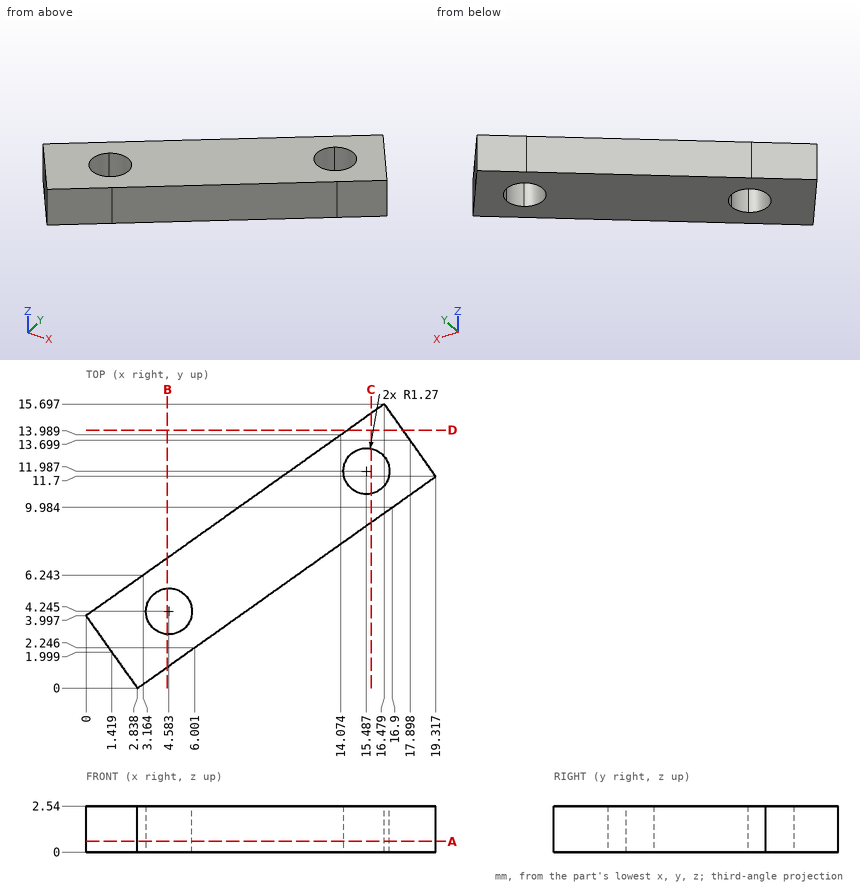
Geometry: see drawing. Coordinates: mm, zero at the bounding-box minimum. Give positions to 0.01 mm unless a question says otherwise; leave off trailing zeros. Loops run counter-clockwise (first coordinate to the right, second up) from the corner with the lowest first, then second, coordinate; pieces in that order, holes last. Notation, with made-up numbers: (-16, -19) - (33, -19) arc R20 ccw to (33, 7) - close; hole circle Ø7 at (31.25, -12). An arc over 180 degrees is marked (long way). Use CSV: the item, a comma, the result in double quotes. Start each with the question number.
1. Pin query (flat end, axial travel): pin 1 (1.5 mm diameter, centred on x = 7, y = 10.5, fed in from -Z); pin 2 (1 mm diameter, centred on x = 11.5, z = 1, fed in from +Y). Return the tip coordinate at first contact, or that it passes through.
2. Section B-B (x = 4.5). Output: boundary loops of the cut face in (y, z).
3. Section D-D (y = 14.25). Output: boundary loops of the cut face in (x, z).
4. Section A-A (z = 0.6). Output: boundary loops of the cut face in (x, y) (1 decimal).
5. Ray query, L1, parallel to X at y = 12.75, z = 0.35 (1 decimal); L2, parallel to Y at x = 3.5, z = 0.45 (1 decimal); L3, parallel to X at y = 6, z = 1.05 (1 decimal). Return the intervals inside material, ascending.
6. Section C-C (x = 15.75). Output: boundary loops of the cut face in (y, z) (1 decimal).
Response:
1,pin 1,"through"
1,pin 2,"y = 12.52"
2,outline,"(1.18, 0) - (2.98, 0) - (2.98, 2.54) - (1.18, 2.54) - close; (5.51, 0) - (7.19, 0) - (7.19, 2.54) - (5.51, 2.54) - close"
3,outline,"(14.44, 0) - (17.51, 0) - (17.51, 2.54) - (14.44, 2.54) - close"
4,outline,"(0, 4) - (2.8, 0) - (19.3, 11.7) - (16.5, 15.7) - close; hole circle Ø2.5 at (4.6, 4.2); hole circle Ø2.5 at (15.5, 12)"
5,L1,"12.3 to 14.5, 16.5 to 18.6"
5,L2,"0.5 to 3.6, 4.9 to 6.5"
5,L3,"2.8 to 11.3"
6,outline,"(9.2, 0) - (10.7, 0) - (10.7, 2.5) - (9.2, 2.5) - close; (13.2, 0) - (15.2, 0) - (15.2, 2.5) - (13.2, 2.5) - close"
